Read the model definition and answer for the solid it produces. Units are mm, in the model's axes. A direction names the side the tool comes from. Coordinates: 2 decimals unless noted, no trailing zeros. Order: outer loops, then holes, each group sorted by start corner. A loop starts at its lowest first (then second) coordinate and runs counter-clockwise, first axis right, second up. Notation, with made-up numbers: M 8.25,81 L 63.25,81 A20 ccw 63.25,100 Z; hole C -21,-30 d2. An arc over 180 degrees is marked long. Put each result on its own line as item: value.
from build123d import *

# Parameters (mm, degrees)
SKETCH_1_W                       = 50
SKETCH_1_H                       = 50
SM_BASE_FLANGE_1_DEPTH           = 2
SM_EDGE_FLANGE_1_STRIP_W         = 10
SM_EDGE_FLANGE_1_STRIP_H         = 2
SM_EDGE_FLANGE_1_STRIP_CUT_DEPTH = 50
SM_EDGE_FLANGE_1_DEPTH           = 50
SKETCH_9_R                       = 15
SKETCH_9_R_2                     = 1.65
CUT_EXTRUDE_2_DEPTH              = 10
SKETCH_12_R                      = 5
SKETCH_12_R_2                    = 2
CUT_EXTRUDE_4_DEPTH              = 10


# Sheet-metal steps are written as plain solids
with BuildPart() as part:
    # Sketch 1 → 基体-法兰1 (new body)
    with BuildSketch(Plane.XY):
        Rectangle(SKETCH_1_W, SKETCH_1_H)
    extrude(amount=-SM_BASE_FLANGE_1_DEPTH)

    # 边线-法兰1 strip (across the edge) → 边线-法兰1 strip cut (cut)
    with BuildSketch(Plane(origin=(-25, 25, -2), x_dir=(0, -1, 0), z_dir=(1, 0, 0))):
        with Locations((-2, -1)):
            Rectangle(SM_EDGE_FLANGE_1_STRIP_W, SM_EDGE_FLANGE_1_STRIP_H)
    extrude(amount=SM_EDGE_FLANGE_1_STRIP_CUT_DEPTH, mode=Mode.SUBTRACT)

    # 边线-法兰1 section (across the edge) → 边线-法兰1 (add)
    with BuildSketch(Plane(origin=(-25, 25, -2), x_dir=(0, -1, 0), z_dir=(1, 0, 0))):
        with BuildLine():
            Line((0, 1), (0, 48))
            Line((0, 48), (2, 48))
            Line((2, 48), (2, 1))
            ThreePointArc((2, 1), (2.292893219, 0.292893219), (3, 0))
            Line((3, 0), (3, -2))
            ThreePointArc((3, -2), (0.878679656, -1.121320344), (0, 1))
        make_face()
    extrude(amount=SM_EDGE_FLANGE_1_DEPTH)

    # 草图9 → 切除-拉伸2 (cut)
    with BuildSketch(Plane.XY):
        Circle(SKETCH_9_R)
        with Locations((-15.202795796, 15.202795796)):
            Circle(SKETCH_9_R_2)
        with Locations((15.202795796, 15.202795796)):
            Circle(SKETCH_9_R_2)
        with Locations((15.202795796, -15.202795796)):
            Circle(SKETCH_9_R_2)
        with Locations((-15.202795796, -15.202795796)):
            Circle(SKETCH_9_R_2)
    extrude(amount=-CUT_EXTRUDE_2_DEPTH, mode=Mode.SUBTRACT)

    # 草图12 → 切除-拉伸4 (cut)
    with BuildSketch(Plane(origin=(0, 25, 0), x_dir=(1, 0, 0), z_dir=(0, 1, 0))):
        with Locations(Location((0, 28, 0), (0, 0, 270))):
            Circle(SKETCH_12_R)
        with Locations(Location((0, 45, 0), (0, 0, 270))):
            Circle(SKETCH_12_R_2)
        with Locations(Location((17, 28, 0), (0, 0, 270))):
            Circle(SKETCH_12_R_2)
        with Locations(Location((0, 11, 0), (0, 0, 270))):
            Circle(SKETCH_12_R_2)
        with Locations(Location((-17, 28, 0), (0, 0, 270))):
            Circle(SKETCH_12_R_2)
    extrude(amount=-CUT_EXTRUDE_4_DEPTH, mode=Mode.SUBTRACT)


solid = part.part
Q1. Find section D-D on z = -45. Write down the section's boundary in (x, y), plus the area to 3 significant figures.
Answers below:
outline: M -25,23 L -2,23 L -2,25 L -25,25 Z; M 2,23 L 25,23 L 25,25 L 2,25 Z
area: 92.0 mm^2
Q2. Find section B-B on z = -28. Write down the section's boundary in (x, y).
Answers below:
outline: M -25,23 L -19,23 L -19,25 L -25,25 Z; M -15,23 L -5,23 L -5,25 L -15,25 Z; M 5,23 L 15,23 L 15,25 L 5,25 Z; M 19,23 L 25,23 L 25,25 L 19,25 Z
Q3. Find section A-A on x = 0. Write down the section's boundary in (y, z).
Answers below:
outline: M -25,-2 L -15,-2 L -15,0 L -25,0 Z; M 15,-2 L 22,-2 A1 cw 23,-3 L 23,-9 L 25,-9 L 25,-3 A3 ccw 22,0 L 15,0 Z; M 23,-50 L 25,-50 L 25,-47 L 23,-47 Z; M 23,-43 L 25,-43 L 25,-33 L 23,-33 Z; M 23,-23 L 25,-23 L 25,-13 L 23,-13 Z
Q4. Consider line 1 along X through (y, z) = (24.5, -28); line 2 along Y through (x, z) = (21, -3); line 3 along Z through (x, y) = (10, 13.5). Determine where each line is inside the solid, lowest interval first.
Answers below:
line 1: x = -25 to -19, -15 to -5, 5 to 15, 19 to 25
line 2: y = 23 to 25
line 3: z = -2 to 0
Q5. Given pin 1 (23.5 mm diameter, centred on x = 9, z = -17, fed in from -Y); pin 2 (10 mm diameter, centred on x = 15.5, y = 9, fed in from -Z), each flat-ended and moving along its own axis, determine where each tip first touches the part or whether it passes through.
Answers below:
pin 1: stops at y = 23
pin 2: stops at z = -2
Q6. Find section C-C on y = 6. Write down the section's boundary in (x, z).
Answers below:
outline: M -25,-2 L -13.75,-2 L -13.75,0 L -25,0 Z; M 13.75,-2 L 25,-2 L 25,0 L 13.75,0 Z
Q7. For a pull along Y with two mould halves and no side action, classify faces 3 (the face through (-14.985, 0.66, -0.986)), 4 (the face through (0, -25, -1)), 5 (the face through (-1.2, 24, -12.6)) as +Y half, -Y half, draft (parallel to the pull), parting line (faces both ways), or undercut.
Answers below:
face 3: undercut
face 4: -Y half
face 5: draft
Q8. A tool of negligible diameter and unlimited length cuts with its end or side. For faces 1 (the face through (-11, -12, -2)), 2 (the face through (13.554, 15.275, -0.986)), from which of +Z, -Z, +X, -X, +Y, -Y can it reach the whole face along a straight path? Write none if from no direction.
Answers below:
face 1: -Z, +X, -X, -Y
face 2: +Z, -Z
